```python
from build123d import *

# Parameters (mm, degrees)
SKETCH1_W           = 50
SKETCH1_H           = 130
BOSS_EXTRUDE1_DEPTH = 16
CUT_EXTRUDE1_DEPTH  = 167


with BuildPart() as part:
    # Sketch1 → Boss-Extrude1 (new body)
    with BuildSketch(Plane(origin=(0, 0, 0), x_dir=(1, 0, 0), z_dir=(0, 1, 0))):
        with Locations((25, -65)):
            Rectangle(SKETCH1_W, SKETCH1_H)
    extrude(amount=BOSS_EXTRUDE1_DEPTH)

    # Sketch3 → Cut-Extrude1 (cut)
    with BuildSketch(Plane.XY.offset(130)):
        Polygon((22.5, 0), (27.5, 0), (26.661208671, 11.995274858), (23.338791329, 11.995274858), align=None)
    extrude(amount=-CUT_EXTRUDE1_DEPTH, mode=Mode.SUBTRACT)


solid = part.part
```
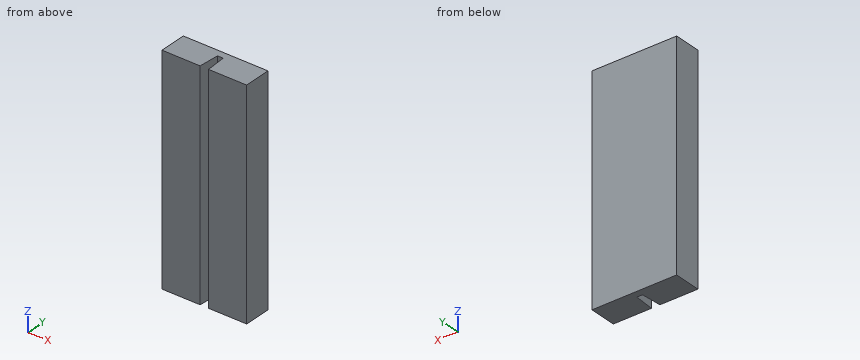
Check sheet for the modelled part. Datum: model origin and axes. Units: mm. Coordinates: 2 decimals unless noted, no trailing zeros. Write each loop counter-clockwise with the first axis right and the second up, starting at its lowest first coordinate (ties: lowest second). Pieces come first, ordered by that corner, then holes. Notation, with made-up numbers: M 25,-34 L 46,-34 A12 ccw 46,-19 Z; hole C 85,-22 d10. An arc over 180 degrees is marked long. Write item = value, one per line. Start each with the question number.
1. Sectioned sample at B-B (z = 25). Record the cut outline in (x, y).
2. Thickness scan on probe 1 along X at (y, z) = (11.75, 91); probe 2 along X at (y, z) = (2.75, 14); probe 3 along Y at (x, z) = (25, 110). Record the ranges inside material, lowest first.
3. Sectioned sample at A-A (y = 10.25). Record the cut outline in (x, z).
The answers:
q1.outline = M 0,0 L 22.5,0 L 23.34,12 L 26.66,12 L 27.5,0 L 50,0 L 50,16 L 0,16 Z
q2.probe_1 = 0 to 23.32, 26.68 to 50
q2.probe_2 = 0 to 22.69, 27.31 to 50
q2.probe_3 = 12 to 16
q3.outline = M 0,0 L 23.22,0 L 23.22,130 L 0,130 Z; M 26.78,0 L 50,0 L 50,130 L 26.78,130 Z
